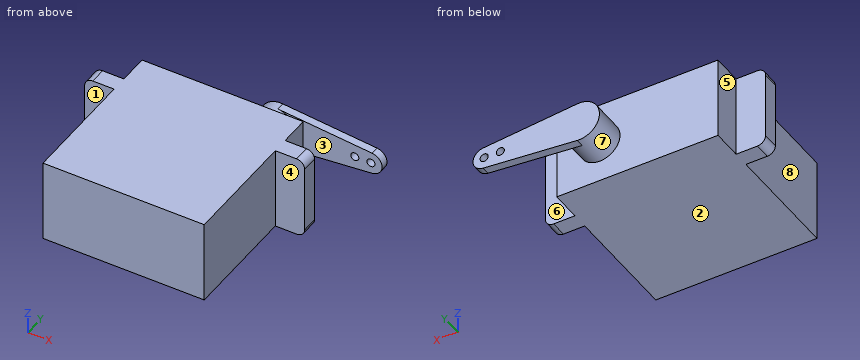
```python
from build123d import *

# Parameters (mm, degrees)
SKETCH2_W           = 39.85
SKETCH2_H           = 20.5
BOSS_EXTRUDE1_DEPTH = 40.4
BOSS_EXTRUDE2_START = 29
SKETCH3_W           = 54.38
SKETCH3_H           = 20.5
BOSS_EXTRUDE2_DEPTH = 4
FILLET1_R           = 2
SKETCH5_R           = 5
BOSS_EXTRUDE3_DEPTH = 8.4
BOSS_EXTRUDE4_START = -2
BOSS_EXTRUDE4_DEPTH = 2
SKETCH7_R           = 1
CUT_EXTRUDE1_DEPTH  = 2


with BuildPart() as part:
    # Sketch2 → Boss-Extrude1 (new body)
    with BuildSketch(Plane(origin=(0, 0, 0), x_dir=(1, 0, 0), z_dir=(0, 1, 0))):
        with Locations((19.925, 10.25)):
            Rectangle(SKETCH2_W, SKETCH2_H)
    extrude(amount=BOSS_EXTRUDE1_DEPTH)

    # Sketch3 → Boss-Extrude2 (add)
    with BuildSketch(Plane(origin=(0, 0, 0), x_dir=(1, 0, 0), z_dir=(0, 1, 0)).offset(BOSS_EXTRUDE2_START)):
        with Locations((19.925, 10.25)):
            Rectangle(SKETCH3_W, SKETCH3_H)
    extrude(amount=BOSS_EXTRUDE2_DEPTH)

    # Fillet1
    fillet1_edges = [part.edges().sort_by_distance(p)[0] for p in [
        (-7.265, 31, 0),
        (47.115, 31, -20.5),
        (-7.265, 31, -20.5),
        (47.115, 31, 0),
    ]]
    fillet(fillet1_edges, radius=FILLET1_R)

    # Sketch5 → Boss-Extrude3 (add)
    with BuildSketch(Plane(origin=(0, 40.4, 0), x_dir=(1, 0, 0), z_dir=(0, 1, 0))):
        with Locations(Location((29.215, 10.25, 0), (0, 0, 90))):
            Circle(SKETCH5_R)
    extrude(amount=BOSS_EXTRUDE3_DEPTH)

    # Sketch6 → Boss-Extrude4 (add)
    with BuildSketch(Plane(origin=(0, 48.8, 0), x_dir=(1, 0, 0), z_dir=(0, 1, 0)).offset(BOSS_EXTRUDE4_START)):
        with BuildLine():
            Line((29.693723404, 15.227029626), (52.978297872, 12.987366295))
            ThreePointArc((52.978297872, 12.987366295), (55.465, 10.25), (52.978297872, 7.512633705))
            Line((52.978297872, 7.512633705), (29.693723404, 5.272970374))
            ThreePointArc((29.693723404, 5.272970374), (24.215, 10.25), (29.693723404, 15.227029626))
        make_face()
    extrude(amount=BOSS_EXTRUDE4_DEPTH)

    # Sketch7 → Cut-Extrude1 (cut)
    with BuildSketch(Plane(origin=(0, 48.8, 0), x_dir=(1, 0, 0), z_dir=(0, 1, 0))):
        with Locations(Location((52.715, 10.25, 0), (0, 0, 270))):
            Circle(SKETCH7_R)
        with Locations(Location((48.715, 10.25, 0), (0, 0, 270))):
            Circle(SKETCH7_R)
    extrude(amount=-CUT_EXTRUDE1_DEPTH, mode=Mode.SUBTRACT)


solid = part.part
```
The listing builds one solid part. Answer for the finished solid, in the listing's coordinates (mm). Face numbers are marked on the shaded views. A direction names the side the tool comes from. Coordinates: 2 decimals unless noted, no trailing zeros. Loops run counter-clockwise (first coordinate to the right, second up) from the corner with the lowest first, then second, coordinate; pieces in that order, holes last. Notation, with made-up numbers: M 8.25,61.5 L 57.25,61.5 A31 ccw 57.25,98.5 Z; hole C 43.25,-12 d1. An arc over 180 degrees is marked long. Answer as CSV lines item,"result". Start each with the question number.
(1) The part is cut by section B-B (x = 36.5). Give the vertices of the cut face in (y, z).
(2) The mould has two halves that part along Y. Classify the marked faces 1, 2 and 3: pulls with the +Y half, pulls with the -Y half, needs draft (parallel to the pull), parting line crosses it, or undercut.
(3) The part is cut by section C-C (y = 23.5). Give the vertices of the cut face in (x, z), and give its area (3 significant figures).
(4) Find the intervals of material crossed by L1, parallel to X at y = 47.45, z = -10.25 (3 decimals); L2, parallel to Y at x = 23, z = -2.5; L3, parallel to X at y = 31.5, z = -10.5 (3 decimals), in increasing order. Write a range as [from, to].
(5) Given pin 1 (8 mm diameter, centred on x = 45, z = -6, fed in from -Y); pin 2 (12 mm diameter, centred on y = 14.5, z = -11, fed in from +X); pin 3 (4 mm diameter, centred on y = 38, z = -8, fed in from -X), each flat-ended and moving along its own axis, determine where each tip first touches the part or whether it passes through.
(6) The part is cut by section A-A (z = -10.25). Give the vertices of the cut face in (x, y) (3 decimals), and give its area (3 significant figures).
(7) For the marked faces 4, 5, 6, 7 and 8, determine the directions among +Z, -Z, +X, -X, +Y, -Y from which every point of the face is accessible in a straight line to the end or side of a thin tool.
(8) The part is cut by section D-D (x = 28). Give the vertices of the cut face in (y, z).
Determined:
1,outline,"M 0,-20.5 L 40.4,-20.5 L 40.4,0 L 0,0 Z; M 46.8,-14.57 L 48.8,-14.57 L 48.8,-5.93 L 46.8,-5.93 Z"
2,face 1,"pulls with the -Y half"
2,face 2,"needs draft"
2,face 3,"undercut"
3,outline,"M 0,-20.5 L 39.85,-20.5 L 39.85,0 L 0,0 Z"
3,area,"817 mm2"
4,L1,"[24.215, 47.715], [49.715, 51.715], [53.715, 55.465]"
4,L2,"[0, 40.4]"
4,L3,"[-7.265, 47.115]"
5,pin 1,"y = 29"
5,pin 2,"x = 39.85"
5,pin 3,"x = 0"
6,outline,"M -7.265,29 L 0,29 L 0,0 L 39.85,0 L 39.85,29 L 47.115,29 L 47.115,33 L 39.85,33 L 39.85,40.4 L 34.215,40.4 L 34.215,46.8 L 47.715,46.8 L 47.715,48.8 L 24.215,48.8 L 24.215,40.4 L 0,40.4 L 0,33 L -7.265,33 Z; M 49.715,46.8 L 51.715,46.8 L 51.715,48.8 L 49.715,48.8 Z; M 53.715,46.8 L 55.465,46.8 L 55.465,48.8 L 53.715,48.8 Z"
6,area,"1,790 mm2"
7,face 4,"+Z, -Z, +X, -Y"
7,face 5,"+Z, -Z, -X, +Y"
7,face 6,"+Z, -Z, +X"
7,face 7,"none"
7,face 8,"+Z, -Z, -X, -Y"
8,outline,"M 0,-20.5 L 40.4,-20.5 L 40.4,-15.1 L 48.8,-15.1 L 48.8,-5.4 L 40.4,-5.4 L 40.4,0 L 0,0 Z"
